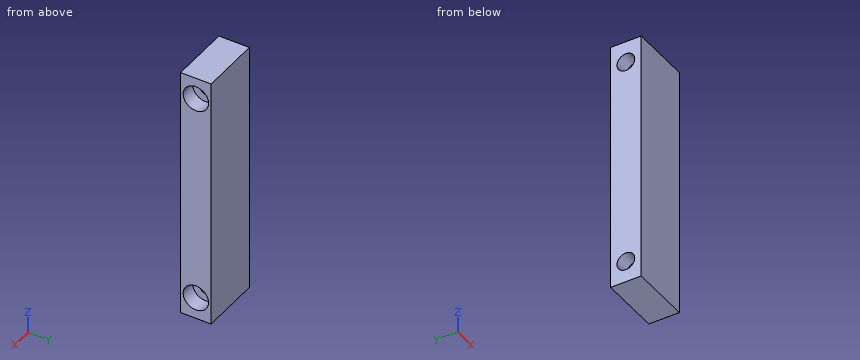
from build123d import *

# Parameters (mm, degrees)
ESQUISSE1_W             = 48
ESQUISSE1_H             = 200
BOSS_EXTRU_1_DEPTH      = 24
ESQUISSE2_R             = 4
ENL_V_MAT_EXTRU_1_DEPTH = 114.490087673
ESQUISSE3_R             = 10
ENL_V_MAT_EXTRU_2_DEPTH = 12
ESQUISSE4_R             = 7
ENL_V_MAT_EXTRU_3_DEPTH = 12


with BuildPart() as part:
    # Esquisse1 → Boss.-Extru.1 (new body)
    with BuildSketch(Plane(origin=(0, 0, 0), x_dir=(1, 0, 0), z_dir=(0, 1, 0))):
        Rectangle(ESQUISSE1_W, ESQUISSE1_H)
    extrude(amount=BOSS_EXTRU_1_DEPTH)

    # Esquisse2 → Enlèv. mat.-Extru.1 (cut, through all)
    with BuildSketch(Plane(origin=(24, 0, 0), x_dir=(0, 0, -1), z_dir=(1, 0, 0))):
        with Locations((-83, 12)):
            Circle(ESQUISSE2_R)
        with Locations((83, 12)):
            Circle(ESQUISSE2_R)
    extrude(amount=-ENL_V_MAT_EXTRU_1_DEPTH, mode=Mode.SUBTRACT)

    # Esquisse3 → Enlèv. mat.-Extru.2 (cut)
    with BuildSketch(Plane(origin=(24, 0, 0), x_dir=(0, 0, -1), z_dir=(1, 0, 0))):
        with Locations((-83, 12)):
            Circle(ESQUISSE3_R)
        with Locations((83, 12)):
            Circle(ESQUISSE3_R)
    extrude(amount=-ENL_V_MAT_EXTRU_2_DEPTH, mode=Mode.SUBTRACT)

    # Esquisse4 → Enlèv. mat.-Extru.3 (cut)
    with BuildSketch(Plane.ZY.offset(24)):
        with Locations((-83, 12)):
            Circle(ESQUISSE4_R)
        with Locations((83, 12)):
            Circle(ESQUISSE4_R)
    extrude(amount=-ENL_V_MAT_EXTRU_3_DEPTH, mode=Mode.SUBTRACT)


solid = part.part
Read the model definition and answer for the solid it produces. Units are mm, in the model's axes. Round coordinates to 2 decimals unless told otherwise and drop trailing zeros. Write each loop counter-clockwise with the first axis right and the second up, starting at its lowest first coordinate (ties: lowest second). Pieces come first, ordered by that corner, then holes. Notation, with made-up numbers: (77, 55.25) - (113, 55.25) arc R8 ccw to (113, 62.25) - close; hole circle Ø1 at (28.5, 42). An arc over 180 degrees is marked (long way). Use a Markdown table: item, result.
(1) The part is cut by section A-A (y = 12). Write down the section's boundary in (x, z).
Reported:
| item | result |
|---|---|
| outline | (-24, -100) - (24, -100) - (24, -93) - (12, -93) - (12, -87) - (-12, -87) - (-12, -90) - (-24, -90) - close; (-24, -76) - (-12, -76) - (-12, -79) - (12, -79) - (12, -73) - (24, -73) - (24, 73) - (12, 73) - (12, 79) - (-12, 79) - (-12, 76) - (-24, 76) - close; (-24, 90) - (-12, 90) - (-12, 87) - (12, 87) - (12, 93) - (24, 93) - (24, 100) - (-24, 100) - close |
(2) The part is cut by section B-B (z = 83). Write down the section's boundary in (x, y), then the cut area to 3 significant figures.
Reported:
| item | result |
|---|---|
| outline | (-24, 0) - (24, 0) - (24, 2) - (12, 2) - (12, 8) - (-12, 8) - (-12, 5) - (-24, 5) - close; (-24, 19) - (-12, 19) - (-12, 16) - (12, 16) - (12, 22) - (24, 22) - (24, 24) - (-24, 24) - close |
| area | 552 mm2 |
(3) The part is cut by section C-C (x = -8). Write down the section's boundary in (y, z), then the cut area to 3 significant figures.
Reported:
| item | result |
|---|---|
| outline | (0, -100) - (24, -100) - (24, 100) - (0, 100) - close; hole circle Ø8 at (12, -83); hole circle Ø8 at (12, 83) |
| area | 4,700 mm2 |
(4) Straight lines are drawn through the part: line 1 along Y through (x, z) = (21, 83); line 2 along Z through (x, y) = (-16, 16); line 3 along Z through (x, y) = (-20, 7.5). For each, find the intervals that lie inside material, in ascending order. Write a range as [from, to].
Reported:
| item | result |
|---|---|
| line 1 | [0, 2], [22, 24] |
| line 2 | [-100, -88.74], [-77.26, 77.26], [88.74, 100] |
| line 3 | [-100, -88.36], [-77.64, 77.64], [88.36, 100] |
(5) Each of these flat-tipped pins is pushed along its axis until it touches: pin 1 Ø12 at (y, z) = (12, -83) entering from -X; pin 2 Ø11 at (y, z) = (12, -83) entering from +X; pin 3 Ø5 at (y, z) = (12, -83) entering from +X. Where does it stop, or does it pass through?
Reported:
| item | result |
|---|---|
| pin 1 | x = -12 |
| pin 2 | x = 12 |
| pin 3 | through |
